Drawing for the job (mm, zero at the part's lowest x, y, z). A direction names the side the tool comes from. Give positions to 0.01 mm unless a question says otherwise; leave off trailing zeros. Order: outer loops, then holes, each group sorted by start corner. A loop starts at its lowest first (then second) coordinate and runs counter-clockwise, first axis right, second up. Notation, with made-up numbers: (65.5, 54) -> (77.5, 54) arc R28 ccw to (77.5, 72) -> close; hole circle Ø4 at (49.25, 44.25). An arc over 180 degrees is marked (long way). One line per item, written item: value. Start each with the question number.
(1) Pin check, flat tips, straight feed: pin 1 (10 mm diameter, centred on y = 20, z = 7, fed in from -X); pin 2 (10 mm diameter, centred on y = 18, z = 10.5, fed in from -X) (1 decimal); pin 3 (10 mm diameter, centred on y = 46.5, z = 9.5, fed in from -X) (1 decimal); pin 4 (10 mm diameter, centred on x = 77, y = 21.5, fed in from +Z). Stop position of each tip, or through.
(2) Saw through at C-C on y = 47. Give the cut face in (x, z) (1 decimal), plus the area to 3 significant figures.
(3) Saw through at A-A on z = 16.25. Give the cut face in (x, y) (1 decimal).
(4) Probe line 1 (X direction, y = 54, z = 1.75) (1 decimal); line 2 (X direction, y = 49, z = 5.75); line 3 (Y direction, x = 94.5, z = 7) (1 decimal). List the from-to ranges inside material, lowest first.
(5) Which spindle directions (+Z, -Z, +X, -X, +Y, -Y) get a long thin tool onto all of the face, cutting with end or side? Do the marked faces 4, 5 and 6. Say none if no direction does.
(6) Saw through at B-B on x = 72. Give the cut face in (y, z) (1 decimal).
(7) Two-plate mould, pull along Y, no slides. Class the marked faces 1, 2 and 3: +Y half, -Y half, draft (parallel to the pull), parting line (faces both ways), or undercut.
(8) Saw through at D-D on y = 26. Give the cut face in (x, z), plus the area to 3 significant figures.
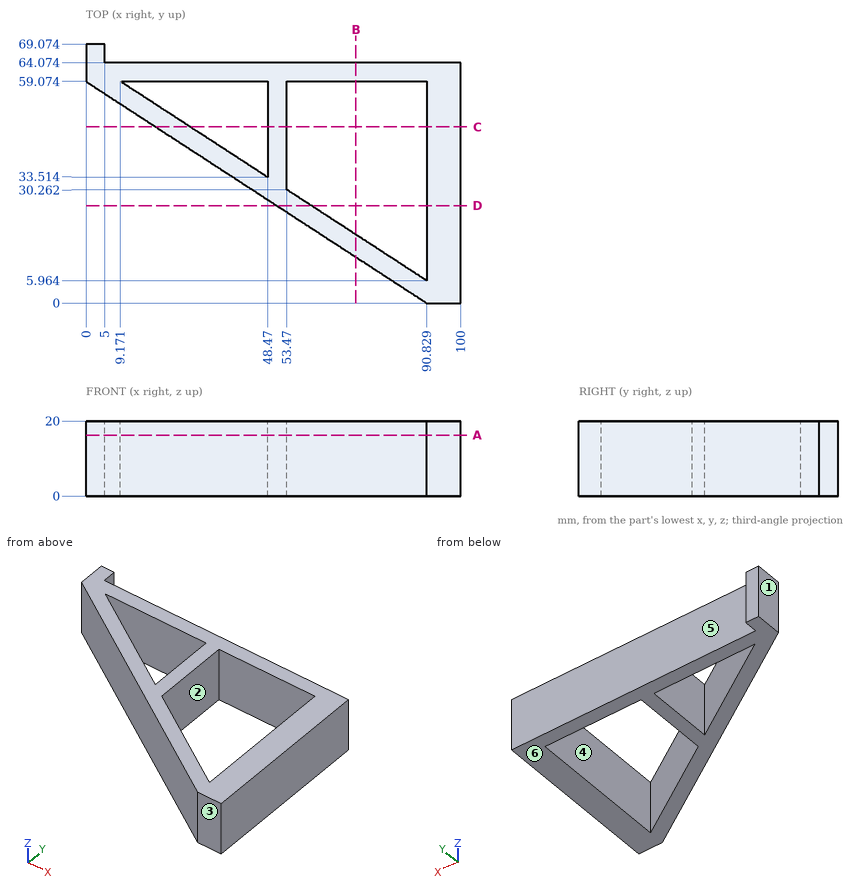
Results below:
1. pin 1: stops at x = 52.39
1. pin 2: stops at x = 55.5
1. pin 3: stops at x = 11.6
1. pin 4: passes through
2. outline: (18.6, 0) -> (27.7, 0) -> (27.7, 20) -> (18.6, 20) -> close; (48.5, 0) -> (53.5, 0) -> (53.5, 20) -> (48.5, 20) -> close; (90.8, 0) -> (100, 0) -> (100, 20) -> (90.8, 20) -> close
2. area: 467 mm²
3. outline: (0, 59.1) -> (90.8, 0) -> (100, 0) -> (100, 64.1) -> (5, 64.1) -> (5, 69.1) -> (0, 69.1) -> close; hole (9.2, 59.1) -> (48.5, 33.5) -> (48.5, 59.1) -> close; hole (53.5, 30.3) -> (90.8, 6) -> (90.8, 59.1) -> (53.5, 59.1) -> close
4. line 1: x = 7.8 to 17, 48.5 to 53.5, 90.8 to 100
4. line 2: x = 15.49 to 24.66, 48.47 to 53.47, 90.83 to 100
4. line 3: y = 0 to 64.1
5. face 4: +Z, -Z
5. face 5: +Z, -Z, +X, +Y
5. face 6: -Z, +X, -X, +Y, -Y
6. outline: (12.2, 0) -> (18.2, 0) -> (18.2, 20) -> (12.2, 20) -> close; (59.1, 0) -> (64.1, 0) -> (64.1, 20) -> (59.1, 20) -> close
7. face 1: draft
7. face 2: undercut
7. face 3: -Y half
8. outline: (50.85, 0) -> (60.02, 0) -> (60.02, 20) -> (50.85, 20) -> close; (90.83, 0) -> (100, 0) -> (100, 20) -> (90.83, 20) -> close
8. area: 367 mm²
